CAD build for the part. Positions are in the model's coordinates, mm. A direction names the side the tool comes from. Give positions to 0.01 mm unless a question says otherwise; leave off trailing zeros. Loops run counter-clockwise (first coordinate to the right, second up) from the corner with the lowest first, then second, coordinate; pieces in that order, holes last. Notation, with made-up numbers: M 61,72 L 92,72 A26 ccw 92,96 Z; hole C -11,16.25 d3. An arc over 180 degrees is marked long. Answer as CSV lines item,"result".
```python
from build123d import *

# Parameters (mm, degrees)
BOSS_EXTRUDE1_DEPTH = 11.43
BOSS_EXTRUDE2_DEPTH = 6.35
SKETCH6_R           = 10.16
BOSS_EXTRUDE3_DEPTH = 13.716
SKETCH7_R           = 10.541
BOSS_EXTRUDE4_DEPTH = 16.51
FILLET1_R           = 1.5875
FILLET2_R           = 1.5875


with BuildPart() as part:
    # Sketch1 → Boss-Extrude1 (new body)
    with BuildSketch(Plane.XY):
        Polygon((14.664696837, 0), (7.332348419, 12.7), (-7.332348419, 12.7), (-14.664696837, 0), (-7.332348419, -12.7), (7.332348419, -12.7), align=None)
    extrude(amount=BOSS_EXTRUDE1_DEPTH)

    # Sketch4 → Boss-Extrude2 (add)
    with BuildSketch(Plane(origin=(-10.998522628, -6.35, 0), x_dir=(0, 0, 1), z_dir=(-0.866025404, -0.5, 0))):
        Polygon((5.715, 0), (5.715, 5.572584798), (0.889, 2.786292399), (0.889, 0), align=None)
        Polygon((5.715, -5.572584798), (5.715, 0), (0.889, 0), (0.889, -2.786292399), align=None)
        Polygon((10.541, 0), (5.715, 0), (5.715, -5.572584798), (10.541, -2.786292399), align=None)
        Polygon((10.541, 2.786292399), (5.715, 5.572584798), (5.715, 0), (10.541, 0), align=None)
    extrude(amount=BOSS_EXTRUDE2_DEPTH)

    # Sketch6 → Boss-Extrude3 (add)
    with BuildSketch(Plane.XY.offset(11.43)):
        Circle(SKETCH6_R)
    extrude(amount=BOSS_EXTRUDE3_DEPTH)

    # Sketch7 → Boss-Extrude4 (add)
    with BuildSketch(Plane(origin=(0, 0, 0), x_dir=(-1, 0, 0), z_dir=(0, 0, -1))):
        Circle(SKETCH7_R)
    extrude(amount=BOSS_EXTRUDE4_DEPTH)

    # Fillet1
    fillet1_edges = [part.edges().sort_by_distance(p)[0] for p in [
        (7.332348419, -12.7, 5.715),
        (-7.332348419, -12.7, 5.715),
        (-14.664696837, 0, 5.715),
        (-7.332348419, 12.7, 5.715),
        (7.332348419, 12.7, 5.715),
        (14.664696837, 0, 5.715),
    ]]
    fillet(fillet1_edges, radius=FILLET1_R)

    # Fillet2
    fillet2_edges = [part.edges().sort_by_distance(p)[0] for p in [
        (-12.355007086, -10.3505, 0.889),
        (-10.961860886, -12.7635, 5.715),
        (-12.355007086, -10.3505, 10.541),
        (-15.141299485, -5.5245, 10.541),
        (-16.534445684, -3.1115, 5.715),
        (-15.141299485, -5.5245, 0.889),
    ]]
    fillet(fillet2_edges, radius=FILLET2_R)


solid = part.part
```
Q1. Cut at D-D (z = 6). Write the cut outline in (x, y) (1 decimal), and give its area (3 significant figures).
Solution:
outline,"M -19.1,-4.9 L -13.8,-14.1 L -8.3,-10.9 L -7.8,-11.9 A1.6 ccw -6.4,-12.7 L 6.4,-12.7 A1.6 ccw 7.8,-11.9 L 14.2,-0.8 A1.6 ccw 14.2,0.8 L 7.8,11.9 A1.6 ccw 6.4,12.7 L -6.4,12.7 A1.6 ccw -7.8,11.9 L -14.2,0.8 A1.6 ccw -14.2,-0.8 L -13.6,-1.8 Z"
area,"625 mm²"
Q2. Pin check, flat tips, straight feed: P1, Ø1.5, axis at x = -12, y = -8, coming from the -Z side; P2, Ø3.5, axis at x = -2.5, z = 4.5, coming from the -Y side; P3, Ø12, axis at y = -4.5, z = -4.5, coming from the +X side. Stop position of each tip, or through.
Solution:
P1,"stops at z = 0.89"
P2,"stops at y = -12.7"
P3,"stops at x = 14.33"
Q3. Cut at C-C (z = 15.5). Write the cut outline in (x, y), and give its area (3 significant figures).
Solution:
outline,"C 0,0 d20.32"
area,"324 mm²"
Q4. Which spindle directions (+Z, -Z, +X, -X, +Y, -Y) get a long thin tool onto all of the face, cutting with end or side? Do faces 1 (the flat face through (-10, 4, 11.43)), 2 (the cylindrical face through (-11.12, -12.57, 5.73)), 3 (the flat face through (-14, -8, 10.541)), 4 (the flat face through (-15.8, -4.3, 3.3)), 5 (the flat face through (-15.793, -4.307, 8.151)). Say none if no direction does.
Solution:
face 1,"+Z"
face 2,"-Y"
face 3,"+Z, -X, -Y"
face 4,"-Z, -X"
face 5,"+Z, -X"
Q5. Cut at A-A (y = 0). Write the cut outline in (x, z).
Solution:
outline,"M -14.42,0 L -10.54,0 L -10.54,-16.51 L 10.54,-16.51 L 10.54,0 L 14.42,0 L 14.42,11.43 L 10.16,11.43 L 10.16,25.15 L -10.16,25.15 L -10.16,11.43 L -14.42,11.43 Z"
Q6. Cut at B-B (x = 0). Write the cut outline in (y, z), and give its area (3 significant figures).
Solution:
outline,"M -12.7,0 L -10.54,0 L -10.54,-16.51 L 10.54,-16.51 L 10.54,0 L 12.7,0 L 12.7,11.43 L 10.16,11.43 L 10.16,25.15 L -10.16,25.15 L -10.16,11.43 L -12.7,11.43 Z"
area,"917 mm²"
Q7. Wall check: line 1 (Z direction, x = -8.5, y = -7); line 2 (Y direction, x = -6.5, z = 5); line 3 (Y direction, x = 0, z = -3). Give the ranges that are in metal, low to high. Write a range as [from, to].
Solution:
line 1,"z = [0, 11.43]"
line 2,"y = [-12.7, 12.7]"
line 3,"y = [-10.54, 10.54]"
Q8. Mould opens along Y. For faces 6 (the flat face through (-13.18, -2.57, 3.09)), 7 (the cylindrical face through (14.42, 0.01, 5.8)), 8 (the flat face through (-14, -8, 0.889)), 9 (the cylindrical face through (-14.42, 0.01, 5.8)) say: released by +Y, released by -Y, zero draft, split by the parting line, or undercut.
Solution:
face 6,"undercut"
face 7,"split by the parting line"
face 8,"zero draft"
face 9,"undercut"
